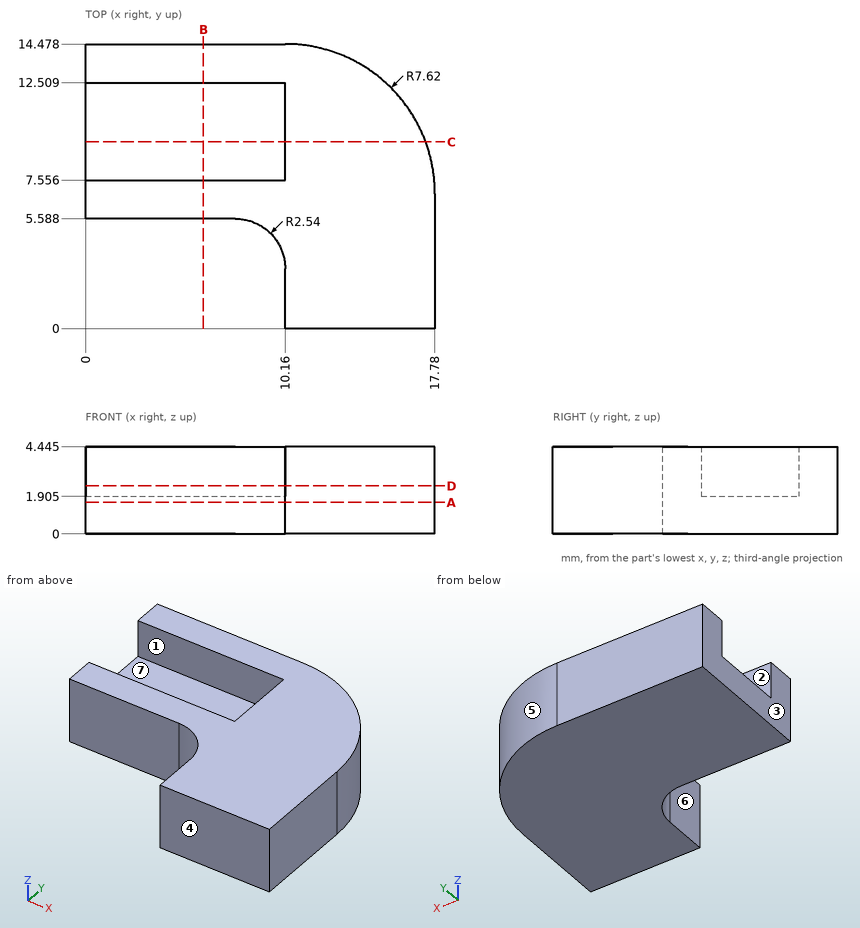
Could you check a few things on this drawing? It's one solid part, dimensions in mm from its lowest x, y, z. A direction names the side the tool comes from. Give positions to 0.01 mm unless a question says otherwise; leave off trailing zeros. Write each loop counter-clockwise with the first axis right and the second up, starting at its lowest first coordinate (ties: lowest second). Pieces come first, ordered by that corner, then holes.
(1) Imagine slicing it at C-C, the plane y = 9.5. Write out the boundary of the cut face in (x, z) (1 decimal).
Output values:
outline: (0, 0) - (17.3, 0) - (17.3, 4.4) - (10.2, 4.4) - (10.2, 1.9) - (0, 1.9) - close
(2) If I drill on L1, parallel to Y at x = 7.75, z = 3.3 (1 decimal); L2, parallel to Z at x = 8, y = 10.75 (1 decimal); L3, parallel to Y at x = 4.75, z = 1.85, over which ranges is the centre line in solid material (lowest first)?
Output values:
L1: y = 5.6 to 7.6, 12.5 to 14.5
L2: z = 0 to 1.9
L3: y = 5.59 to 14.48
(3) Will these pins go through, and if not, where does the flat tip stop? pin 1 (1.5 mm diameter, centred on x = 7, y = 9, fed in from +Z) (1 decimal); pin 2 (1.3 mm diameter, centred on x = 3, z = 2.5, fed in from -Y); pin 3 (2.5 mm diameter, centred on y = 1, z = 1.5, fed in from -X).
Output values:
pin 1: stops at z = 1.9
pin 2: stops at y = 5.59
pin 3: stops at x = 10.16
(4) Thinking about a two-plate mould opening in Y: for the marked faces 1, 2, 3 and 4, which applies, pulls with the +Y half, pulls with the -Y half, needs draft (parallel to the pull), parting line crosses it, or undercut?
Output values:
face 1: undercut
face 2: undercut
face 3: needs draft
face 4: pulls with the -Y half
(5) Imagine slicing it at D-D, the plane z = 2.45. Write out the boundary of the cut face in (x, y).
Output values:
outline: (0, 5.59) - (7.62, 5.59) arc R2.54 cw to (10.16, 3.05) - (10.16, 0) - (17.78, 0) - (17.78, 6.86) arc R7.62 ccw to (10.16, 14.48) - (0, 14.48) - (0, 12.51) - (10.16, 12.51) - (10.16, 7.56) - (0, 7.56) - close
(6) On a 3-axis mill with a long thin cutter (end or side, diameter ignored), from which of +Z, -Z, +X, -X, +Y, -Y can I reach the whole of each face in a straight line? I mean the marked faces 5, 6 and 7. Say none if no direction works.
Output values:
face 5: +Z, -Z, +X, +Y
face 6: +Z, -Z, -X, -Y
face 7: +Z, -X
(7) Imagine slicing it at B-B, the plane x = 6. Write out the boundary of the cut face in (y, z) (1 decimal).
Output values:
outline: (5.6, 0) - (14.5, 0) - (14.5, 4.4) - (12.5, 4.4) - (12.5, 1.9) - (7.6, 1.9) - (7.6, 4.4) - (5.6, 4.4) - close
(8) Imagine slicing it at A-A, the plane z = 1.6. Write out the boundary of the cut face in (x, y).
Output values:
outline: (0, 5.59) - (7.62, 5.59) arc R2.54 cw to (10.16, 3.05) - (10.16, 0) - (17.78, 0) - (17.78, 6.86) arc R7.62 ccw to (10.16, 14.48) - (0, 14.48) - close
